Here's how the part is built. I have some questions about the finished solid (model axes, mm). Face numbers are marked on the shaded views. A direction names the side the tool comes from. Round coordinates to 2 decimals unless told otherwise and drop trailing zeros. Write each loop counter-clockwise with the first axis right and the second up, starting at its lowest first coordinate (ties: lowest second). Pieces come first, ordered by that corner, then holes. Notation, with made-up numbers: (88, 5) -> (131, 5) arc R18 cw to (131, 16) -> close; hole circle Ø7 at (42.5, 44.25). An arc over 180 degrees is marked (long way). Answer in a Markdown table with one row per item.
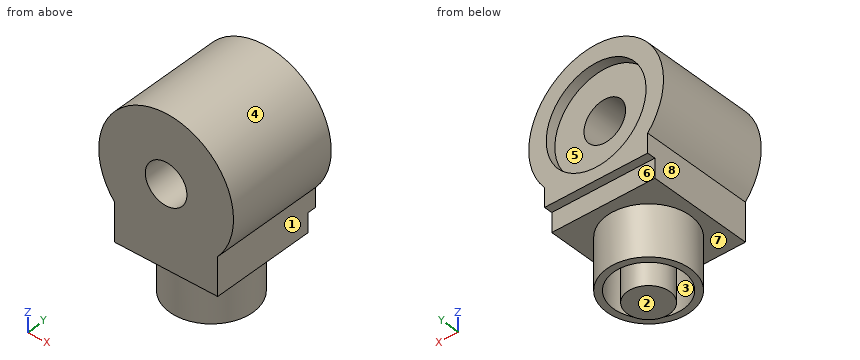
from build123d import *

# Parameters (mm, degrees)
BOSS_EXTRUDE1_DEPTH        = 34.544
SKETCH2_R                  = 15.24
CUT_EXTRUDE1_DEPTH         = 3.048
F_1_2_0_5_DIAMETER_HOLE1_D = 12.7
SKETCH5_W                  = 31.496
SKETCH5_H                  = 5.842
CUT_EXTRUDE2_DEPTH         = 2.54
SKETCH8_R                  = 12.7
SKETCH8_R_2                = 10.668
BOSS_EXTRUDE3_DEPTH        = 15.494
SKETCH9_R                  = 6.477
BOSS_EXTRUDE4_DEPTH        = 19.05
SKETCH6_R                  = 12.7
BOSS_EXTRUDE2_DEPTH        = 15.494
CUT_EXTRUDE3_START         = -15.494
SKETCH7_R                  = 10.668
SKETCH7_R_2                = 6.477
CUT_EXTRUDE3_DEPTH         = 15.494


with BuildPart() as part:
    # Sketch1 → Boss-Extrude1 (new body)
    with BuildSketch(Plane(origin=(0, 0, 0), x_dir=(1, 0, 0), z_dir=(0, 1, 0))):
        with BuildLine():
            Line((15.748, 24.892), (-15.748, 24.892))
            Line((-15.748, 24.892), (-15.748, 13.23971193))
            ThreePointArc((-15.748, 13.23971193), (0, -20.574), (15.748, 13.23971193))
            Line((15.748, 13.23971193), (15.748, 24.892))
        make_face()
    extrude(amount=BOSS_EXTRUDE1_DEPTH)

    # Sketch2 → Cut-Extrude1 (cut)
    with BuildSketch(Plane(origin=(0, 34.544, 0), x_dir=(1, 0, 0), z_dir=(0, 1, 0))):
        with Locations(Location((0, 0, 0), (0, 0, 270))):
            Circle(SKETCH2_R)
    extrude(amount=-CUT_EXTRUDE1_DEPTH, mode=Mode.SUBTRACT)

    # 1/2 (0.5) Diameter Hole1 (through all)
    with Locations(Plane(origin=(0, 31.496, 0), x_dir=(1, 0, 0), z_dir=(0, 1, 0))):
        with Locations((0, 0)):
            Hole(F_1_2_0_5_DIAMETER_HOLE1_D / 2)

    # Sketch5 → Cut-Extrude2 (cut)
    with BuildSketch(Plane(origin=(0, 34.544, 0), x_dir=(1, 0, 0), z_dir=(0, 1, 0))):
        with Locations((0, 21.971)):
            Rectangle(SKETCH5_W, SKETCH5_H)
    extrude(amount=-CUT_EXTRUDE2_DEPTH, mode=Mode.SUBTRACT)

    # Sketch8 → Boss-Extrude3 (add)
    with BuildSketch(Plane(origin=(0, 0, -24.892), x_dir=(-1, 0, 0), z_dir=(0, 0, -1))):
        with Locations(Location((0, 16.002, 0), (0, 0, 180))):
            Circle(SKETCH8_R)
        with Locations((0, 16.002)):
            Circle(SKETCH8_R_2, mode=Mode.SUBTRACT)
    extrude(amount=BOSS_EXTRUDE3_DEPTH)

    # Sketch9 → Boss-Extrude4 (add)
    with BuildSketch(Plane(origin=(0, 0, -24.892), x_dir=(-1, 0, 0), z_dir=(0, 0, -1))):
        with Locations(Location((0, 16.002, 0), (0, 0, 180))):
            Circle(SKETCH9_R)
    extrude(amount=BOSS_EXTRUDE4_DEPTH)

    # Sketch6 → Boss-Extrude2 (add)
    with BuildSketch(Plane(origin=(0, 0, -24.892), x_dir=(-1, 0, 0), z_dir=(0, 0, -1))):
        with Locations(Location((0, 16.002, 0), (0, 0, 180))):
            Circle(SKETCH6_R)
    extrude(amount=BOSS_EXTRUDE2_DEPTH)

    # Sketch7 → Cut-Extrude3 (cut)
    with BuildSketch(Plane(origin=(0, 0, -40.386), x_dir=(-1, 0, 0), z_dir=(0, 0, -1)).offset(CUT_EXTRUDE3_START)):
        with Locations((0, 16.002)):
            Circle(SKETCH7_R)
        with Locations(Location((0, 16.002, 0), (0, 0, 180))):
            Circle(SKETCH7_R_2, mode=Mode.SUBTRACT)
    extrude(amount=CUT_EXTRUDE3_DEPTH, mode=Mode.SUBTRACT)


solid = part.part
1) I want a section at B-B, the plane z = 0. List the corners of the cut face in (x, y) for me.
Response:
| item | result |
|---|---|
| outline | (-20.57, 0) -> (-6.35, 0) -> (-6.35, 31.5) -> (-15.24, 31.5) -> (-15.24, 34.54) -> (-20.57, 34.54) -> close; (6.35, 0) -> (20.57, 0) -> (20.57, 34.54) -> (15.24, 34.54) -> (15.24, 31.5) -> (6.35, 31.5) -> close |
2) I need wall thicknesses on line 1 (X direction, y = 33, z = 0); line 2 (Y direction, x = -11, z = -20.5); line 3 (Y direction, x = 8.5, z = 4). Which ranges of each line are inside material? Lowest first, please. Write a range as [from, to].
Response:
| item | result |
|---|---|
| line 1 | x = [-20.57, -15.24], [15.24, 20.57] |
| line 2 | y = [0, 32] |
| line 3 | y = [0, 31.5] |
3) I want a section at A-A, the plane x = 0. List the corners of the cut face in (y, z) for me (3 decimals).
Response:
| item | result |
|---|---|
| outline | (0, -24.892) -> (3.302, -24.892) -> (3.302, -40.386) -> (5.334, -40.386) -> (5.334, -24.892) -> (9.525, -24.892) -> (9.525, -43.942) -> (22.479, -43.942) -> (22.479, -24.892) -> (26.67, -24.892) -> (26.67, -40.386) -> (28.702, -40.386) -> (28.702, -24.892) -> (32.004, -24.892) -> (32.004, -19.05) -> (34.544, -19.05) -> (34.544, -15.24) -> (31.496, -15.24) -> (31.496, -6.35) -> (0, -6.35) -> close; (0, 6.35) -> (31.496, 6.35) -> (31.496, 15.24) -> (34.544, 15.24) -> (34.544, 20.574) -> (0, 20.574) -> close |
4) We'd pull the mould along X, two halves only. Please class the marked faces 1, 2 and 3: +X half, -X half, draft (parallel to the pull), parting line (faces both ways), or undercut.
Response:
| item | result |
|---|---|
| face 1 | +X half |
| face 2 | draft |
| face 3 | undercut |
5) I want a section at D-D, the plane x = 12. List the corners of the cut face in (y, z) for me.
Response:
| item | result |
|---|---|
| outline | (0, -24.89) -> (11.84, -24.89) -> (11.84, -40.39) -> (20.16, -40.39) -> (20.16, -24.89) -> (32, -24.89) -> (32, -19.05) -> (34.54, -19.05) -> (34.54, -9.39) -> (31.5, -9.39) -> (31.5, 9.39) -> (34.54, 9.39) -> (34.54, 16.71) -> (0, 16.71) -> close |
6) I want a section at C-C, the plane y = 11. List the corners of the cut face in (x, z) for me.
Response:
| item | result |
|---|---|
| outline | (-15.75, -24.89) -> (-11.67, -24.89) -> (-11.67, -40.39) -> (-9.42, -40.39) -> (-9.42, -24.89) -> (-4.11, -24.89) -> (-4.11, -43.94) -> (4.11, -43.94) -> (4.11, -24.89) -> (9.42, -24.89) -> (9.42, -40.39) -> (11.67, -40.39) -> (11.67, -24.89) -> (15.75, -24.89) -> (15.75, -13.24) arc R20.57 ccw (long way) to (-15.75, -13.24) -> close; hole circle Ø12.7 at (0, 0) |
7) Which directions (+Z, -Z, +X, -X, +Y, -Y) give clear straight access to the entire face, cutting with the end or side of a thin tool? Please do the marked faces 4, 5, 6, 7 and 8.
Response:
| item | result |
|---|---|
| face 4 | +Y, -Y |
| face 5 | +Y |
| face 6 | -Z, +X, -X, +Y |
| face 7 | -Z |
| face 8 | -Z, -X, +Y, -Y |
8) For pin 1 (12 mm diameter, centred on x = -13, y = 24.5, fed in from -Z); pin 2 (3 mm diameter, centred on x = -8, y = 34, fed in from -Z); pin 3 (12 mm diameter, centred on y = 9, z = -24.5, fed in from -X), each with a flat end and sliding along its axis, tell me the tip position at first contact or that it passes through.
Response:
| item | result |
|---|---|
| pin 1 | stops at z = -40.39 |
| pin 2 | stops at z = -19.05 |
| pin 3 | stops at x = -15.75 |
